from build123d import *

# Parameters (mm, degrees)
ESBO_O1_R                = 2.1
ESBO_O1_R_2              = 4.5
RESSALTO_EXTRUS_O1_DEPTH = 15
ESBO_O2_R                = 2.1
CORTE_EXTRUS_O1_DEPTH    = 15
CORTE_EXTRUS_O2_DEPTH    = 3
ESBO_O5_R                = 11.25
CORTE_EXTRUS_O3_DEPTH    = 10
FILETE1_R                = 5


with BuildPart() as part:
    # Esboço1 → Ressalto-extrusão1 (new body)
    with BuildSketch(Plane.XY):
        with BuildLine():
            Line((-30.310889132, 77.5), (-82.27241336, -12.5))
            ThreePointArc((-82.27241336, -12.5), (-82.27241336, -47.5), (-51.961524227, -65))
            Line((-51.961524227, -65), (51.961524227, -65))
            ThreePointArc((51.961524227, -65), (82.27241336, -47.5), (82.27241336, -12.5))
            Line((82.27241336, -12.5), (30.310889132, 77.5))
            ThreePointArc((30.310889132, 77.5), (0, 95), (-30.310889132, 77.5))
        make_face()
        with Locations((-12, 70)):
            Circle(ESBO_O1_R, mode=Mode.SUBTRACT)
        with Locations((-66.621778265, -24.607695155)):
            Circle(ESBO_O1_R, mode=Mode.SUBTRACT)
        with Locations(Location((12, 70, 0), (0, 0, 180))):
            Circle(ESBO_O1_R, mode=Mode.SUBTRACT)
        with Locations(Location((-54.621778265, -45.392304845, 0), (0, 0, 180))):
            Circle(ESBO_O1_R, mode=Mode.SUBTRACT)
        with Locations((66.621778265, -24.607695155)):
            Circle(ESBO_O1_R, mode=Mode.SUBTRACT)
        with Locations((54.621778265, -45.392304845)):
            Circle(ESBO_O1_R, mode=Mode.SUBTRACT)
        with Locations((25.980762114, -15)):
            Circle(ESBO_O1_R_2, mode=Mode.SUBTRACT)
    extrude(amount=RESSALTO_EXTRUS_O1_DEPTH)

    # Esboço2 → Corte-extrusão1 (cut)
    with BuildSketch(Plane(origin=(0, 0, 0), x_dir=(-1, 0, 0), z_dir=(0, 0, -1))):
        with Locations((38.97114317, 22.5)):
            Circle(ESBO_O2_R)
        with Locations((41.889318689, -16.440346096)):
            Circle(ESBO_O2_R)
        with Locations((13.263982849, -43.00077626)):
            Circle(ESBO_O2_R)
        with Locations((-25.349402613, -37.180744844)):
            Circle(ESBO_O2_R)
        with Locations((-44.874170873, -3.362854211)):
            Circle(ESBO_O2_R)
        with Locations((-30.6077732, 32.987334232)):
            Circle(ESBO_O2_R)
        with Locations((6.706901978, 44.49738718)):
            Circle(ESBO_O2_R)
    extrude(amount=-CORTE_EXTRUS_O1_DEPTH, mode=Mode.SUBTRACT)

    # Esboço4 → Corte-extrusão2 (cut)
    with BuildSketch(Plane(origin=(0, 0, 0), x_dir=(-1, 0, 0), z_dir=(0, 0, -1))):
        with BuildLine():
            Line((51.961524227, -65), (-51.961524227, -65))
            ThreePointArc((-51.961524227, -65), (-82.27241336, -47.5), (-82.27241336, -12.5))
            Line((-82.27241336, -12.5), (-30.310889132, 77.5))
            ThreePointArc((-30.310889132, 77.5), (0, 95), (30.310889132, 77.5))
            Line((30.310889132, 77.5), (82.27241336, -12.5))
            ThreePointArc((82.27241336, -12.5), (82.27241336, -47.5), (51.961524227, -65))
        make_face()
        with BuildLine():
            Line((51.961524227, -61.5), (-51.961524227, -61.5))
            ThreePointArc((-51.961524227, -61.5), (-79.241324446, -45.75), (-79.241324446, -14.25))
            Line((-79.241324446, -14.25), (-27.279800219, 75.75))
            ThreePointArc((-27.279800219, 75.75), (0, 91.5), (27.279800219, 75.75))
            Line((27.279800219, 75.75), (79.241324446, -14.25))
            ThreePointArc((79.241324446, -14.25), (79.241324446, -45.75), (51.961524227, -61.5))
        make_face(mode=Mode.SUBTRACT)
    extrude(amount=-CORTE_EXTRUS_O2_DEPTH, mode=Mode.SUBTRACT)

    # Esboço5 → Corte-extrusão3 (cut)
    with BuildSketch(Plane.XY.offset(15)):
        with Locations((25.980762114, -15)):
            Circle(ESBO_O5_R)
    extrude(amount=-CORTE_EXTRUS_O3_DEPTH, mode=Mode.SUBTRACT)

    # Filete1
    filete1_edges = [part.edges().sort_by_distance(p)[0] for p in [
        (-82.27241336, -47.5, 15),
        (0, -65, 15),
        (82.27241336, -47.5, 15),
        (56.291651246, 32.5, 15),
        (0, 95, 15),
        (-56.291651246, 32.5, 15),
    ]]
    fillet(filete1_edges, radius=FILETE1_R)


solid = part.part
The model under review builds one solid part; all positions refer to its coordinate system, in mm. A direction names the side the tool comes from. Give positions to 0.01 mm unless a question says otherwise; leave off trailing zeros. One line per question, with ' | ' between items. Start each with the question number.
Item 1: We need section A-A on z = 12. Give the number of separate pieces and of enclosed holes in the cut face, plus the area to 3 significant figures.
Item 2: For faces 4 (the cylindrical face through (0.462, 91.497, 1.479)), 5 (the cylindrical face through (1, -64, 13)), list the 3-axis set-ups (+Z, -Z, +X, -X, +Y, -Y) from which the entire face can be reached by the end or side of a thin tool; tool diameter is ignored.
Item 3: Draft analysis for pull direction X (two halves, no side actions). For faces 1 (the cylindrical face through (79.007, -46.148, 1.479)), 2 (the flat face through (31, -15, 5)), 3 (the cylindrical face through (-55.421, 31.157, 13.496)), state which applies: released by +X, released by -X, zero draft, split by the parting line, or undercut.
Item 4: For pin 1 (1.5 mm diameter, centred on x = -20, z = 1, fed in from -Y); pin 2 (1 mm diameter, centred on y = 13, z = 13.5, fed in from -X); pin 3 (18 mm diameter, centred on x = 25.98, y = -15, fed in from +Z), all flat-tipped, find the tip position at first contact; note any pin that passes through.
Item 5: Wall thickness on line 1 (Y direction, x = 12, z = 4.25); line 2 (X direction, y = 43, z = 1.75); line 3 (Y direction, x = -68, z = 12): over which ranges is each line inside the solid? List them lowest first. Write a range as from..to.
Results found:
1) separate pieces: 1 | enclosed holes: 14 | area: 18,600 mm2
2) face 4: -Z, +Y | face 5: +Z, +X, -X, -Y
3) face 1: released by +X | face 2: undercut | face 3: released by -X
4) pin 1: stops at y = -61.5 | pin 2: stops at x = -66.48 | pin 3: stops at z = 5
5) line 1: y = -65..67.9, 72.1..92.88 | line 2: x = -46.19..-8.18, -5.23..46.19 | line 3: y = -60.64..-26.19, -23.02..11.39
